Autodesk Inventor part; units mm, degrees
ref_plane "YZ Plane" through (0, 0, 0) normal (1, 0, 0) x (0, 1, 0)
ref_plane "XZ Plane" through (0, 0, 0) normal (0, 1, 0) x (-1, 0, 0)
ref_plane "XY Plane" through (0, 0, 0) normal (0, 0, 1) x (1, 0, 0)
sketch "Sketch1" plane through (0, 0, 0) normal (0, 0, 1) x (1, 0, 0)
  line L0 (0, 38.1) -> (0, 0)
  line L1 (0, 0) -> (127, 0)
  line L2 (127, 0) -> (127, 38.1)
  arc A0 (0, 38.1) -> (25.4, 63.5) centre (0, 63.5) ccw
  arc A1 (101.6, 63.5) -> (127, 38.1) centre (127, 63.5) ccw
  line L3 (25.4, 101.6) -> (25.4, 63.5)
  line L4 (25.4, 101.6) -> (38.1, 101.6)
  line L5 (38.1, 101.6) -> (38.1, 88.9)
  line L6 (38.1, 88.9) -> (88.9, 88.9)
  line L7 (88.9, 88.9) -> (88.9, 101.6)
  line L8 (88.9, 101.6) -> (101.6, 101.6)
  line L9 (101.6, 101.6) -> (101.6, 63.5)
  arc A2 (38.1, 33.3375) -> (38.1, 17.4625) centre (38.1, 25.4) ccw
  arc A3 (88.9, 17.4625) -> (88.9, 33.3375) centre (88.9, 25.4) ccw
  line L10 (88.9, 33.3375) -> (38.1, 33.3375)
  line L11 (38.1, 17.4625) -> (88.9, 17.4625)
extrude "Extrusion1" add sketch "Sketch1" along normal blind 31.75
properties part number "P2-5"
Input: part model. Units: mm. Frame: model coordinates. A direction names the side the tool comes from. Give positions to 0.01 mm unless a question says otherwise; leave off trailing zeros. Order: outer loops, then holes, each group sorted by start corner. A loop starts at its lowest first (then second) coordinate and runs counter-clockwise, first axis right, second up. Notation, with made-up numbers: (-28, 54) -> (11, 54) arc R22 ccw to (11, 75) -> close; hole circle Ø1 at (35.25, 22.25). An arc over 180 degrees is marked (long way). Use one line per item in the form item = value.
1) First-contact query: pin 1 Ø12 at (x, z) = (68, 12.5) entering from +Y; pin 2 Ø4 at (y, z) = (97.5, 11.5) entering from +X; pin 3 Ø9.5 at (y, z) = (82, 8) entering from -X. Flat tips, straight axial feed; report the tip coordinate or a pass-through.
Response values:
pin_1 = 88.9
pin_2 = 101.6
pin_3 = 25.4
2) Section A-A, the plane x = 51.5. Return loops of the section in (y, z), and give its area (3 significant figures).
Response values:
outline = (0, 0) -> (17.46, 0) -> (17.46, 31.75) -> (0, 31.75) -> close; (33.34, 0) -> (88.9, 0) -> (88.9, 31.75) -> (33.34, 31.75) -> close
area = 2,320 mm^2
3) Section B-B, the plane y = 28.5. Return loops of the section in (x, z).
Response values:
outline = (0, 0) -> (30.79, 0) -> (30.79, 31.75) -> (0, 31.75) -> close; (96.21, 0) -> (127, 0) -> (127, 31.75) -> (96.21, 31.75) -> close
4) Line query: probe 1 along Y at (x, z) = (81.5, 11); probe 2 along Y at (x, z) = (89.5, 10.5); probe 3 along X at (y, z) = (92, 21). Output: solid intervals per line, ascending.
Response values:
probe_1 = 0 to 17.46, 33.34 to 88.9
probe_2 = 0 to 17.49, 33.31 to 101.6
probe_3 = 25.4 to 38.1, 88.9 to 101.6
5) Mould query, pull axis X, two halves, no side actions, for faces 5 (the flat face through (127, 19, 16)), 6 (the flat face through (63, 40, 31.75)), 7 (the flat face through (63, 17.462, 16)). Classes: pulls with the +X half, pulls with the -X half, needs draft (parallel to the pull), parting line crosses it, or undercut.
Response values:
face_5 = pulls with the +X half
face_6 = needs draft
face_7 = undercut
6) Reachability of faces 1 (the flat face through (25.4, 83, 16)), 2 (the flat face through (64, 33.338, 16)), 3 (the flat face through (101.6, 83, 16)), 4 (the flat face through (38.1, 95, 16)) from +Z, -Z, +X, -X, +Y, -Y: full face, straight path, thin tool, end or side. Return the list, or none.
Response values:
face_1 = +Z, -Z, -X, +Y
face_2 = +Z, -Z
face_3 = +Z, -Z, +X, +Y
face_4 = +Z, -Z, +Y
7) Section D-D, the plane y = 67.5. Return loops of the section in (x, z), and give its area (3 significant figures).
Response values:
outline = (25.4, 0) -> (101.6, 0) -> (101.6, 31.75) -> (25.4, 31.75) -> close
area = 2,420 mm^2
8) Section C-C, the plane z = 6. Return loops of the section in (x, y) (1 decimal).
Response values:
outline = (0, 0) -> (127, 0) -> (127, 38.1) arc R25.4 cw to (101.6, 63.5) -> (101.6, 101.6) -> (88.9, 101.6) -> (88.9, 88.9) -> (38.1, 88.9) -> (38.1, 101.6) -> (25.4, 101.6) -> (25.4, 63.5) arc R25.4 cw to (0, 38.1) -> close; hole (38.1, 17.5) -> (88.9, 17.5) arc R7.9 ccw to (88.9, 33.3) -> (38.1, 33.3) arc R7.9 ccw to start
